```python
from build123d import *

# Parameters (mm, degrees)
F1_DEPTH       = 25.4
F2_D           = 6.7564
F2_CSINK_D     = 13.4874
F2_CSINK_ANGLE = 82
F4_W           = 63.5
F4_H           = 6.35
F1_FACE_W      = 63.5
F1_FACE_H      = 25.4
F7_D           = 31.75


with BuildPart() as f1:
    # F0 (on Top) → F1 (new body)
    with BuildSketch(Plane.XY):
        Polygon((0.1623489741, 63.8174524204), (-25.2376510259, 63.8174524204), (-25.2376510259, 0.3174524204), (-12.5376510259, 0.3174524204), (0.1623489741, 0.3174524204), align=None)
    extrude(amount=F1_DEPTH)

    # F2 (through all)
    with Locations(Plane(origin=(0, 0, 0), x_dir=(1, 0, 0), z_dir=(0, 0, -1))):
        with Locations((-12.5376510259, -11.7474524204), (-12.5376510259, -32.0674524204), (-12.5376510259, -52.3874524204)):
            CounterSinkHole(F2_D / 2, F2_CSINK_D / 2, counter_sink_angle=F2_CSINK_ANGLE)

    # F4 (on offset) → F5 section 0
    with BuildSketch(Plane.YZ.offset(25.4)):
        with Locations((31.75, 22.3743102956)):
            Rectangle(F4_W, F4_H)
    # F1_face (on face) → F5 section 1
    with BuildSketch(Plane(origin=(0.1623489741, 32.0674524204, 12.7), x_dir=(0, 1, 0), z_dir=(1, 0, 0))):
        Rectangle(F1_FACE_W, F1_FACE_H)
    loft()

    # F7 (through all)
    with Locations(Plane(origin=(-0.1502598385, 0, 25.3981505524), x_dir=(0.9999824999, 0, 0.0059160689), z_dir=(-0.0059160689, 0, 0.9999824999))):
        with Locations((25.9500681529, 31.75)):
            Hole(F7_D / 2)


solid = f1.part
```
CAD build for the part. Positions are in the model's coordinates, mm. A direction names the side the tool comes from. Round coordinates to 2 decimals unless told otherwise and drop trailing zeros. Use a Markdown table: item, result. Add a question column.
(1) Pull direction Y, two halves, no side cores. Call faces 1 (the face through (-12, 63.817, 13)), 2 (the face through (-11.77, 55.845, 3.684)), 3 (the face through (-11.77, 15.205, 3.684)), 4 (the face through (-13, 0.317, 13)): +Y half, -Y half, draft (parallel to the pull), parting line (faces both ways), or undercut.
(2) Flat gauge pins, fed straight in: pin 1 (4 mm diameter, centred on x = 14, z = 17, fed in from -Y); pin 2 (10 mm diameter, centred on x = -18, z = 13, fed in from -Y); pin 3 (11 mm diameter, centred on x = -12.54, y = 11.75, fed in from +Z); pin 4 (6 mm diameter, centred on x = -12.54, y = 32.07, fed in from +Z). Where does each tip first touch, or does it go through?
(3) Cut at A-A (x = -11). State how many separate pieces and enclosed holes the cut face has, and give its area (3 significant figures).
(4) Which spindle directions (+Z, -Z, +X, -X, +Y, -Y) get a long thin tool onto all of the face, cutting with end or side? Do faces 5 (the face through (-12.098, 28.718, 14.786)), 6 (the face through (-18, 33, 25.4)), 7 (the face through (9.97, 31.41, 18.35)). Say none if no direction does.
(5) Drill centre lines: line 1 (Y direction, x = -20.5, z = 21.75); line 2 (Z direction, x = -18, y = 24.5); line 3 (Y direction, x = 18, z = 20). Where is each one in solid material? Low to high.
Geometry says:
| question | item | result |
|---|---|---|
| 1 | face 1 | +Y half |
| 1 | face 2 | undercut |
| 1 | face 3 | undercut |
| 1 | face 4 | -Y half |
| 2 | pin 1 | stops at y = 0.12 |
| 2 | pin 2 | stops at y = 0.32 |
| 2 | pin 3 | stops at z = 25.4 |
| 2 | pin 4 | passes through |
| 3 | separate pieces | 4 |
| 3 | enclosed holes | 0 |
| 3 | area | 1,110 mm² |
| 4 | face 5 | +Z, -Z |
| 4 | face 6 | +Z, -X, +Y, -Y |
| 4 | face 7 | +Z, +X |
| 5 | line 1 | y = 0.32 to 63.82 |
| 5 | line 2 | z = 0 to 25.4 |
| 5 | line 3 | y = 0.09 to 17.94, 45.56 to 63.59 |
